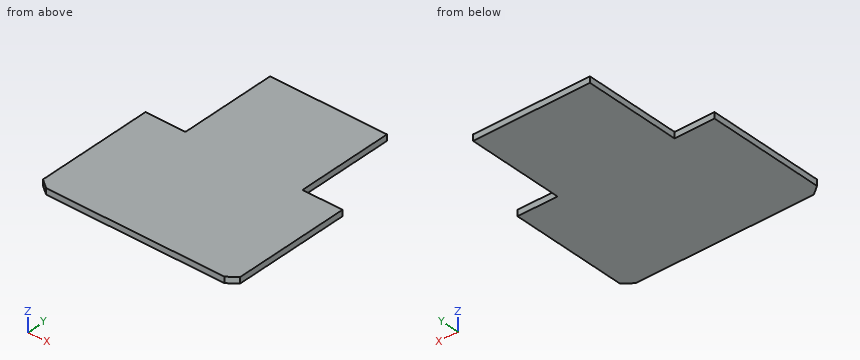
```python
from build123d import *

# Parameters (mm, degrees)
PAD094_DEPTH = 10
SKETCH228_W  = 195.239
SKETCH228_H  = 162.3575
PAD117_DEPTH = 10


with BuildPart() as part:
    # Sketch187 → Pad094 (new body)
    with BuildSketch(Plane(origin=(0, 0, 0), x_dir=(-1, 0, 0), z_dir=(0, 0, -1))):
        Polygon((0, 97.7066), (164.4, 97.7066), (164.4, -99.195429), (148.790353, -111.193448), (0, -111.193448), align=None)
    pad094 = extrude(amount=PAD094_DEPTH)

    # Mirrored033: Pad094 across Sketch187 V_Axis
    add(pad094.mirror(Plane(origin=(0, 0, 0), x_dir=(0, 0, -1), z_dir=(-1, 0, 0))))

    # Sketch228 → Pad117 (join)
    with BuildSketch(Plane(origin=(0, 0, 0), x_dir=(-1, 0, 0), z_dir=(0, 0, -1))):
        with Locations((0, 178.88535)):
            Rectangle(SKETCH228_W, SKETCH228_H)
    extrude(amount=PAD117_DEPTH)


with BuildPart() as part_1:
    # Body072 placement: moved
    add(part.part.moved(Location((0, 0, -5))))


solid = part_1.part
```
Source: CAD feature listing. Evaluate the final solid. Frame: model axes, mm. Give positions to 0.01 mm unless a question says otherwise; leave off trailing zeros. Write each loop counter-clockwise with the first axis right and the second up, starting at its lowest first coordinate (ties: lowest second). Pieces come first, ordered by that corner, then holes.
1. Material intervals for line 1 along X through (y, z) = (202, -10.5); line 2 along Y through (x, z) = (-140.5, -6.5), sorted ascending.
2. Section query C-C (y = 177). Return the cut outline in (x, z).
3. First-contact query: pin 1 (3 mm diameter, centred on y = 147.5, z = -8.5, fed in from +X); pin 2 (5 mm diameter, centred on x = -145.5, z = -11.5, fed in from +Y); pin 3 (5 mm diameter, centred on y = 197.5, z = -7.5, fed in from -X). Flat tips, straight axial feed; report the tip coordinate or a pass-through.
4. Section query A-A (z = -7.5). Return the cut outline in (x, y).
5. Section query B-B (x = -137). Return the cut outline in (y, z), then the cut area to 3 significant figures.
Output values:
1. line 1: x = -97.62 to 97.62
1. line 2: y = -111.19 to 97.71
2. outline: (-97.62, -15) - (97.62, -15) - (97.62, -5) - (-97.62, -5) - close
3. pin 1: stops at x = 97.62
3. pin 2: stops at y = 97.71
3. pin 3: stops at x = -97.62
4. outline: (-164.4, -99.2) - (-148.79, -111.19) - (148.79, -111.19) - (164.4, -99.2) - (164.4, 97.71) - (97.62, 97.71) - (97.62, 260.06) - (-97.62, 260.06) - (-97.62, 97.71) - (-164.4, 97.71) - close
5. outline: (-111.19, -15) - (97.71, -15) - (97.71, -5) - (-111.19, -5) - close
5. area: 2,090 mm2
